Model file for the job. Use its own axes, mm. A direction names the side the tool comes from. Give positions to 0.01 mm unless a question says otherwise; leave off trailing zeros. Loops run counter-clockwise (first coordinate to the right, second up) from the corner with the lowest first, then second, coordinate; pieces in that order, holes last. Notation, with made-up numbers: (33, 69.25) - (57, 69.25) arc R17 cw to (57, 80.25) - close; hole circle Ø5 at (26, 55). An arc over 180 degrees is marked (long way). Use a Markdown table: item, result.
from build123d import *

# Parameters (mm, degrees)
CROQUIS1_R              = 2.1
SALIENTE_EXTRUIR1_DEPTH = 10


with BuildPart() as part:
    # Croquis1 → Saliente-Extruir1 (new body)
    with BuildSketch(Plane.XY):
        with BuildLine():
            Line((-3.244321048, 35), (0, 35))
            Line((0, 35), (0, -5))
            Line((0, -5), (-3.01811075, -5))
            ThreePointArc((-3.01811075, -5), (-11.269152373, -12.457471031), (-19, -4.462))
            Line((-19, -4.462), (-19, 33.038))
            ThreePointArc((-19, 33.038), (-11.988576853, 40.976684766), (-3.244321048, 35))
        make_face()
        with Locations((-11, -4.462)):
            Circle(CROQUIS1_R, mode=Mode.SUBTRACT)
        with Locations((-11, 33.038)):
            Circle(CROQUIS1_R, mode=Mode.SUBTRACT)
    extrude(amount=SALIENTE_EXTRUIR1_DEPTH)


solid = part.part
(1) Drill centre lines: probe 1 along Y at (x, z) = (-11, 2.75); probe 2 along Y at (x, z) = (-12.75, 3.75); probe 3 along Y at (x, z) = (-1.5, 4.75). Where is each one in solid material? Low to high. Write a range as [from, to].
Computed:
| item | result |
|---|---|
| probe 1 | [-12.46, -6.56], [-2.36, 30.94], [35.14, 41.04] |
| probe 2 | [-12.27, -5.62], [-3.3, 31.88], [34.2, 40.84] |
| probe 3 | [-5, 35] |
(2) Pin check, flat tips, straight feed: P1, Ø1.5, axis at x = -14, z = 4, coming from the +Y side; P2, Ø3.5, axis at x = -1, z = 3, coming from the -Y side; P3, Ø6, axis at x = -6.5, z = 8, coming from the +Y side. Stop position of each tip, or through.
Computed:
| item | result |
|---|---|
| P1 | y = 40.72 |
| P2 | y = -5 |
| P3 | y = 40.9 |
(3) Slice it at D-D, the plane x = -6. Write the cut outline in (y, z), plus the area to 3 significant figures.
Computed:
| item | result |
|---|---|
| outline | (-10.71, 0) - (39.28, 0) - (39.28, 10) - (-10.71, 10) - close |
| area | 500 mm² |
(4) Slice it at A-A, the plane z = 3.5. Write the cut outline in (x, y).
Computed:
| item | result |
|---|---|
| outline | (-19, -4.46) arc R8 ccw to (-3.02, -5) - (0, -5) - (0, 35) - (-3.24, 35) arc R8 ccw to (-19, 33.04) - close; hole circle Ø4.2 at (-11, -4.46); hole circle Ø4.2 at (-11, 33.04) |
(5) Mould opens along Y. For faces 1 (the flat face through (-19, 14, 5)), 2 (the flat face through (-1, -5, 5)), 3 (the cylindrical face through (-13.1, -4.4, 4.9)) say: pulls with the +Y half, pulls with the -Y half, needs draft (parallel to the pull), parting line crosses it, or undercut.
Computed:
| item | result |
|---|---|
| face 1 | needs draft |
| face 2 | pulls with the -Y half |
| face 3 | undercut |
(6) Slice it at B-B, the plane x = -11. Write the cut outline in (y, z).
Computed:
| item | result |
|---|---|
| outline | (-12.46, 0) - (-6.56, 0) - (-6.56, 10) - (-12.46, 10) - close; (-2.36, 0) - (30.94, 0) - (30.94, 10) - (-2.36, 10) - close; (35.14, 0) - (41.04, 0) - (41.04, 10) - (35.14, 10) - close |
(7) Slice it at C-C, the plane y = 33.5. Write the cut outline in (x, z), plus the area to 3 significant figures.
Computed:
| item | result |
|---|---|
| outline | (-18.99, 0) - (-13.05, 0) - (-13.05, 10) - (-18.99, 10) - close; (-8.95, 0) - (0, 0) - (0, 10) - (-8.95, 10) - close |
| area | 149 mm² |
(8) 3-axis set-ups, long thin cutter, end or side, ignore diameter. For faces 4 (the flat face through (-2, 35, 5)), 5 (the flat face through (0, 15, 5)): which of +Z, -Z, +X, -X, +Y, -Y reach the whole face in a straight line?
Computed:
| item | result |
|---|---|
| face 4 | +Z, -Z, +X, +Y |
| face 5 | +Z, -Z, +X, +Y, -Y |
